Could you check a few things on this model? Use its own coordinates, in mm. Face numbers are marked on the shaded views. A direction names the side the tool comes from. Coordinates: 2 decimals unless noted, no trailing zeros. Order: outer loops, then holes, each group sorted by start corner. A loop starts at its lowest first (then second) coordinate and runs counter-clockwise, first axis right, second up. Notation, with made-up numbers: (-36, 9) -> (19, 9) arc R25 ccw to (19, 46) -> close; hole circle Ø6 at (-38.75, 52.25). An arc over 180 degrees is marked (long way). Use a Markdown table: item, result. Add a question column.
1) If we section it at B-B (x = 22.5): Write out the boundary of the cut face in (y, z), plus the area to 3 significant figures.
2) If we section it at D-D (z = -6): Write out the boundary of the cut face in (x, y), plus the area to 3 significant figures.
3) If I drill on L1, parallel to Y at x = -22.5, z = -6.5; L2, parallel to Y at x = 21, z = -6; L3, parallel to X at y = 0.6, z = 1.25, over which ranges is the centre line in solid material (lowest first)? Write a range as [from, to].
4) If we section it at A-A (z = 3): Write out the boundary of the cut face in (x, y).
5) Will these pins go through, and if not, where does the flat tip stop? pin 1 Ø1 at (x, y) = (4.5, -0.5) entering from +Z; pin 2 Ø2 at (y, z) = (-0.5, 9) entering from +X; pin 3 Ø2 at (x, z) = (-21, 8) entering from -Y.
6) If we section it at C-C (y = 0.7): Write out the boundary of the cut face in (x, z), plus the area to 3 significant figures.
7) Which directions (+Z, -Z, +X, -X, +Y, -Y) give clear straight access to the entire face, cutting with the end or side of a thin tool? Please do the marked faces 1, 2, 3 and 4.
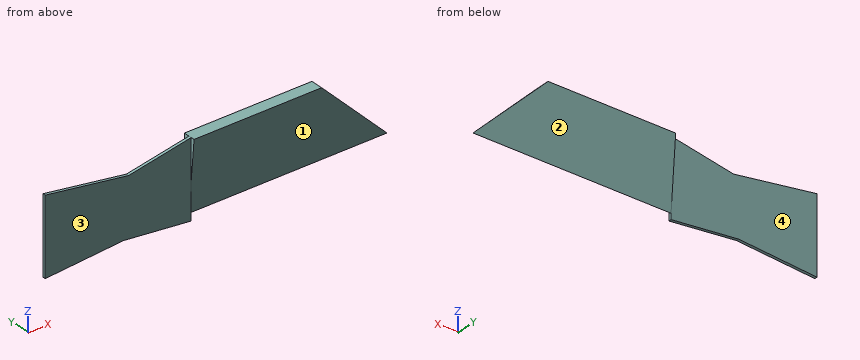
```python
from build123d import *

# Parameters (mm, degrees)
F1_DEPTH    = 59.944
F2_T1_DEPTH = 133.9811516914
F4_DEPTH    = 0.762


# Not quite as in the source:
# - a fillet or chamfer that OpenCascade refuses, or shapes differently, is made with other operations: its cross-section is extruded or revolved along the edge and cut away or added


with BuildPart() as f1:
    # F0 (on Right) → F1 (new body)
    with BuildSketch(Plane.YZ):
        Polygon((1.5876128762, 10.7069341466), (0, 10.7069341466), (-1.7520430265, 10.7069341466), (0, -8.3708763123), align=None)
    extrude(amount=F1_DEPTH)

    # F2: chamfer of 25.4 on 1 edges, made by hand

    # F2_s2 → F2_t1 (cut)
    with BuildSketch(Plane.XZ.offset(-66.9083607706)):
        Polygon((59.944, -14.6930658534), (34.544, 10.7069341466), (59.944, 10.7069341466), align=None)
    extrude(amount=F2_T1_DEPTH, mode=Mode.SUBTRACT)

    # F3 (on Front) → F4 (join)
    with BuildSketch(Plane.XZ):
        Polygon((0, -9.9282488227), (0, 10.7069341466), (-16.936423257, 7.592190057), (-39.5183227956, 11.0962782055), (-39.5183227956, -9.5389056951), (-18.2991251349, -7.9815322533), align=None)
    extrude(amount=F4_DEPTH)


solid = f1.part
```
Answer sheet:
| question | item | result |
|---|---|---|
| 1 | outline | (-1.75, 10.71) -> (0, -8.37) -> (1.59, 10.71) -> close |
| 1 | area | 31.9 mm2 |
| 2 | outline | (-39.52, -0.76) -> (0, -0.76) -> (0, -0.22) -> (51.25, -0.22) -> (51.25, 0.2) -> (0, 0.2) -> (0, 0) -> (-39.52, 0) -> close |
| 2 | area | 51.4 mm2 |
| 3 | L1 | [-0.76, 0] |
| 3 | L2 | [-0.22, 0.2] |
| 3 | L3 | [0, 44] |
| 4 | outline | (-39.52, -0.76) -> (0, -0.76) -> (0, -1.04) -> (42.25, -1.04) -> (42.25, 0.95) -> (0, 0.95) -> (0, 0) -> (-39.52, 0) -> close |
| 5 | pin 1 | z = 10.71 |
| 5 | pin 2 | x = 37.25 |
| 5 | pin 3 | y = -0.76 |
| 6 | outline | (0, 0.04) -> (45.21, 0.04) -> (34.54, 10.71) -> (0, 10.71) -> close |
| 6 | area | 425 mm2 |
| 7 | face 1 | -Z, +X, -Y |
| 7 | face 2 | -Z, +X, -X, +Y |
| 7 | face 3 | +Z, -Z, -X, -Y |
| 7 | face 4 | +Z, -Z, -X, +Y |
